Geometry check sheet. Reference: the model listing, model coordinates, mm. A direction names the side the tool comes from. Coordinates: 2 decimals unless noted, no trailing zeros. Write each loop counter-clockwise with the first axis right and the second up, starting at its lowest first coordinate (ties: lowest second). Pieces come first, ordered by that corner, then holes. Notation, with made-up numbers: M 75,81.25 L 118,81.25 A30 ccw 118,119.25 Z; hole C 67,-17.75 d5. An arc over 180 degrees is marked long. Write item = value, one per line. Start each with the question number.
```python
from build123d import *

# Parameters (mm, degrees)
CYLINDER003_R           = 1.5
CYLINDER003_DEPTH       = 6
CYLINDER003_ROLL_ANGLE  = 90
CYLINDER002_R           = 30
CYLINDER002_DEPTH       = 20
CYLINDER001_R           = 29
CYLINDER001_DEPTH       = 32
CYLINDER001_PITCH_ANGLE = 90
CYLINDER_R              = 29
CYLINDER_DEPTH          = 60
SKETCH_R                = 27.4
POCKET_DEPTH            = 58
SKETCH002_R             = 2.6
SKETCH002_R_2           = 3
POCKET002_DEPTH         = 6
SKETCH001_R             = 1.7
POCKET003_DEPTH         = 5
SKETCH003_W             = 2
SKETCH003_H             = 4.5
SKETCH003_W_2           = 4.5
SKETCH003_H_2           = 2
PAD_DEPTH               = 34
CHAMFER_SIZE            = 2
CHAMFER001_SIZE         = 1


with BuildPart() as cylinder003:
    # Cylinder003 → Cylinder003 (new body)
    with BuildSketch(Plane.XY):
        Circle(CYLINDER003_R)
    extrude(amount=CYLINDER003_DEPTH)


with BuildPart() as cylinder003_1:
    # Cylinder003 roll: moved
    add(cylinder003.part.rotate(Axis((0, 0, 0), (1, 0, 0)), CYLINDER003_ROLL_ANGLE))


with BuildPart() as cylinder003_2:
    # Cylinder003 placement: moved
    add(cylinder003_1.part.moved(Location((0, 30, 46))))


with BuildPart() as cylinder002:
    # Cylinder002 → Cylinder002 (new body)
    with BuildSketch(Plane.XY.offset(50)):
        Circle(CYLINDER002_R)
    extrude(amount=CYLINDER002_DEPTH)


with BuildPart() as cylinder001:
    # Cylinder001 → Cylinder001 (new body)
    with BuildSketch(Plane.XY):
        Circle(CYLINDER001_R)
    extrude(amount=CYLINDER001_DEPTH)


with BuildPart() as cylinder001_1:
    # Cylinder001 pitch: moved
    add(cylinder001.part.rotate(Axis((0, 0, 0), (0, 1, 0)), CYLINDER001_PITCH_ANGLE))


with BuildPart() as cylinder001_2:
    # Cylinder001 placement: moved
    add(cylinder001_1.part.moved(Location((0, 0, 30))))


with BuildPart() as cut:
    # Cylinder → Cylinder (new body)
    with BuildSketch(Plane.XY):
        Circle(CYLINDER_R)
    extrude(amount=CYLINDER_DEPTH)

    # Fusion: union Cylinder001
    add(cylinder001_2.part)

    # Sketch → Pocket (cut)
    with BuildSketch(Plane.XY.offset(60)):
        Circle(SKETCH_R)
    extrude(amount=-POCKET_DEPTH, mode=Mode.SUBTRACT)

    # Sketch002 → Pocket002 (cut)
    with BuildSketch(Plane.YZ.offset(32)):
        with Locations((0, 30)):
            Circle(SKETCH002_R)
        with Locations((0, 44)):
            Circle(SKETCH002_R_2)
        with Locations((0, 16)):
            Circle(SKETCH002_R_2)
    extrude(amount=-POCKET002_DEPTH, mode=Mode.SUBTRACT)

    # Sketch001 → Pocket003 (cut)
    with BuildSketch(Plane.XY.offset(2)):
        with Locations((-15.5, 15.5)):
            Circle(SKETCH001_R)
        with Locations((15.5, 15.5)):
            Circle(SKETCH001_R)
        with Locations((-15.5, -15.5)):
            Circle(SKETCH001_R)
        with Locations((15.5, -15.5)):
            Circle(SKETCH001_R)
    extrude(amount=-POCKET003_DEPTH, mode=Mode.SUBTRACT)

    # Cut: cut Cylinder002
    add(cylinder002.part, mode=Mode.SUBTRACT)


with BuildPart() as cut001:
    # Sketch003 → Pad (new body)
    with BuildSketch(Plane.XY):
        with Locations((-11, 23.45)):
            Rectangle(SKETCH003_W, SKETCH003_H)
        with Locations((11, 23.45)):
            Rectangle(SKETCH003_W, SKETCH003_H)
        with Locations((-11, -23.45)):
            Rectangle(SKETCH003_W, SKETCH003_H)
        with Locations((11, -23.45)):
            Rectangle(SKETCH003_W, SKETCH003_H)
        with Locations((-23.45, 11)):
            Rectangle(SKETCH003_W_2, SKETCH003_H_2)
        with Locations((-23.45, -11)):
            Rectangle(SKETCH003_W_2, SKETCH003_H_2)
        with Locations((23.45, 11)):
            Rectangle(SKETCH003_W_2, SKETCH003_H_2)
        with Locations((23.45, -11)):
            Rectangle(SKETCH003_W_2, SKETCH003_H_2)
    extrude(amount=PAD_DEPTH)

    # Chamfer
    chamfer_edges = [cut001.edges().sort_by_distance(p)[0] for p in [
        (-21.2, -11, 34),
        (-11, -21.2, 34),
        (-21.2, 11, 34),
        (-11, 21.2, 34),
        (11, -21.2, 34),
        (21.2, -11, 34),
        (21.2, 11, 34),
        (11, 21.2, 34),
    ]]
    chamfer(chamfer_edges, length=CHAMFER_SIZE)

    # Fusion001: union Cut
    add(cut.part)

    # Chamfer001
    chamfer001_edges = [cut001.edges().sort_by_distance(p)[0] for p in [
        (-29, 0, 0),
    ]]
    chamfer(chamfer001_edges, length=CHAMFER001_SIZE)

    # Cut001: cut Cylinder003
    add(cylinder003_2.part, mode=Mode.SUBTRACT)


solid = cut001.part
```
Q1. Set-up check for faces 1 (the face through (-10, -23, 18)), 2 (the face through (17.07, 14.85, 1.01)), 3 (the face through (29.67, 1.4, 32.19)): record each of +Z, -Z, +X, -X, +Y, -Y from which the full face is reachable in a straight line by a thin tool's end or side.
Q2. Cross-section at B-B on y = 15.5. Count the separate pieces of the cut face and the enclosed holes in it, and give its area (3 significant figures).
Q3. Scan lines: L1, parallel to Y at x = 29.05, z = 30; L2, parallel to Y at x = 22, z = 24.5; L3, parallel to Y at x = -15.5, z = 1.55. Record each from-to range of solid material in increasing order.
Q4. Draft check along X on faces 4 (the face through (17.07, -16.15, 1.01)), 5 (the face through (11, -21.2, 17)), 6 (the face through (29.65, -0.65, 13.07)). Enter one of: pulls with the +X half, pulls with the -X half, needs draft (parallel to the pull), parting line crosses it, or undercut.
Q5. Cross-section at A-A on z = 46. Enter the section's corners in (x, y).
Q6. Gauge pin test, flat ends, axial feed: pin 1 (10 mm diameter, centred on x = 7.5, y = 0, fed in from -Z); pin 2 (6 mm diameter, centred on x = -14.5, y = 15, fed in from +Z); pin 3 (4.5 mm diameter, centred on x = -23, z = 11, fed in from +Y); pin 4 (2 mm diameter, centred on y = 11.5, z = 15, fed in from -X). Record the tip position at first contact, or that the pin passes through.
Q7. Cross-section at C-C on z = 36. Enter the section's corners in (x, y).
Values found:
q1.face_1 = +Z
q1.face_2 = +Z, -Z
q1.face_3 = +X
q2.separate_pieces = 3
q2.enclosed_holes = 0
q2.area = 629 mm²
q3.L1 = -29 to -2.6, 2.6 to 29
q3.L2 = -28.47 to -16.33, -12 to -10, 10 to 12, 16.33 to 28.47
q3.L3 = -24.51 to -17.2, -13.8 to 13.8, 17.2 to 24.51
q4.face_4 = undercut
q4.face_5 = undercut
q4.face_6 = needs draft
q5.outline = M -1.5,27.36 L -1.5,28.96 A29 ccw long 16,-24.19 L 32,-24.19 L 32,-2.24 L 27.31,-2.24 A27.4 cw long Z; M 1.5,27.36 A27.4 cw 27.31,2.24 L 32,2.24 L 32,24.19 L 16,24.19 A29 ccw 1.5,28.96 Z
q6.pin_1 = 0
q6.pin_2 = 2
q6.pin_3 = 20.26
q6.pin_4 = -27.03
q7.outline = M 6,-28.37 L 32,-28.37 L 32,28.37 L 6,28.37 A29 ccw long Z; hole C 0,0 d54.8
